Check sheet for the drawn part. Datum: minimum x, y, z corner. Units: mm. Give positions to 0.01 mm unless a question says otherwise; leave off trailing zeros. Order: outer loops, then holes, each group sorted by start corner. A loop starts at its lowest first (then second) coordinate and runs counter-clockwise, first axis right, second up. Notation, with made-up numbers: (58, -14) -> (69, -14) arc R21 ccw to (69, -7) -> close; hole circle Ø7 at (55.25, 84). An arc over 180 degrees is marked (long way). Answer in a Markdown table with one row per item. Add a question column.
(1) Thickness scan on L1, parallel to Z at x = 1.9, y = 56.22; L2, parallel to Z at x = 2.95, y = 15; L3, parallel to Y at x = 3.8, z = 18.5 (1 decimal). Record the ranges inside material, lowest first. Write a range as [from, to].
(2) Cross-section at D-D (y = 24). Record the cut outline in (x, z).
(3) Cross-section at C-C (z = 103.25). Record the cut outline in (x, y), then the cut area to 3 significant figures.
(4) Cross-section at B-B (y = 65). Record the cut outline in (x, z).
(5) Cross-section at A-A (z = 16.6). Record the cut outline in (x, y).
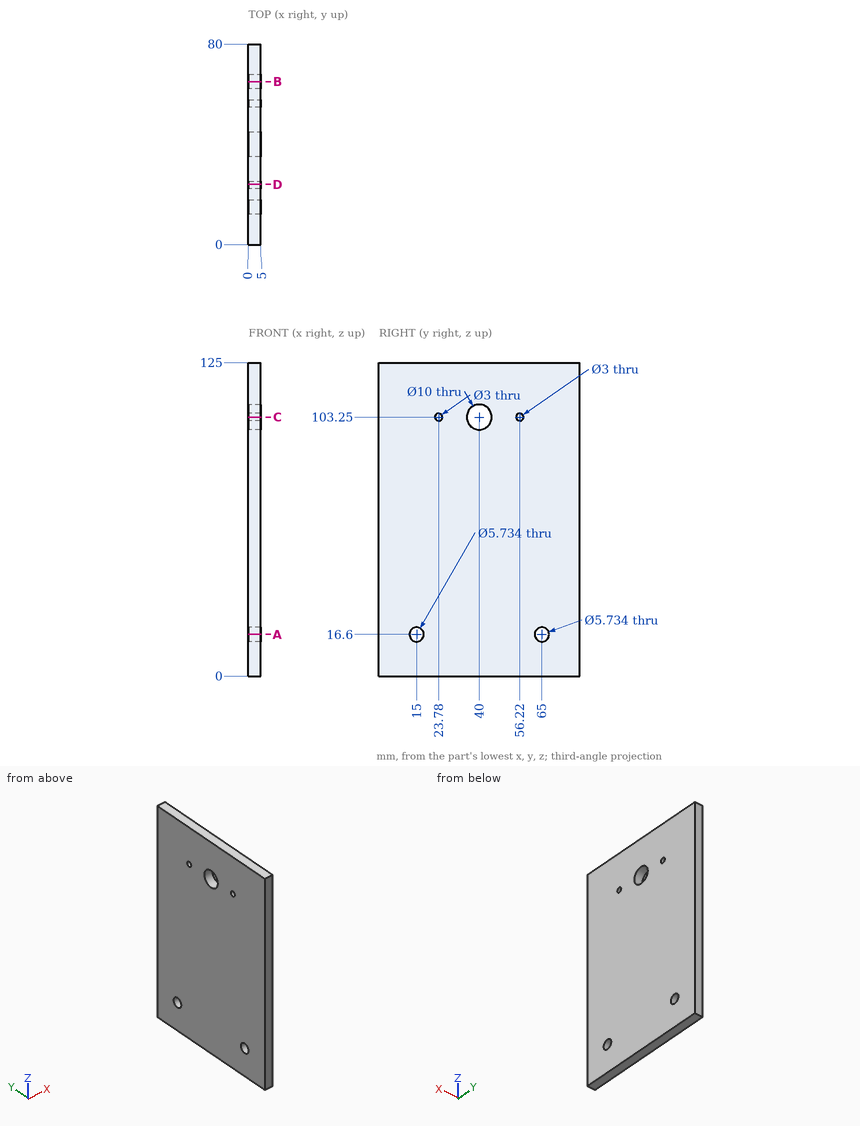
Answer below:
| question | item | result |
|---|---|---|
| 1 | L1 | z = [0, 101.75], [104.75, 125] |
| 1 | L2 | z = [0, 13.73], [19.47, 125] |
| 1 | L3 | y = [0, 12.9], [17.1, 62.9], [67.1, 80] |
| 2 | outline | (0, 0) -> (5, 0) -> (5, 101.77) -> (0, 101.77) -> close; (0, 104.73) -> (5, 104.73) -> (5, 125) -> (0, 125) -> close |
| 3 | outline | (0, 0) -> (5, 0) -> (5, 22.28) -> (0, 22.28) -> close; (0, 25.28) -> (5, 25.28) -> (5, 35) -> (0, 35) -> close; (0, 45) -> (5, 45) -> (5, 54.72) -> (0, 54.72) -> close; (0, 57.72) -> (5, 57.72) -> (5, 80) -> (0, 80) -> close |
| 3 | area | 320 mm² |
| 4 | outline | (0, 0) -> (5, 0) -> (5, 13.73) -> (0, 13.73) -> close; (0, 19.47) -> (5, 19.47) -> (5, 125) -> (0, 125) -> close |
| 5 | outline | (0, 0) -> (5, 0) -> (5, 12.13) -> (0, 12.13) -> close; (0, 17.87) -> (5, 17.87) -> (5, 62.13) -> (0, 62.13) -> close; (0, 67.87) -> (5, 67.87) -> (5, 80) -> (0, 80) -> close |
